Here's how the part is built. I have some questions about the finished solid (model axes, mm). Face numbers are marked on the shaded views. A direction names the side the tool comes from. Round coordinates to 2 decimals unless told otherwise and drop trailing zeros. Write each loop counter-clockwise with the first axis right and the second up, starting at its lowest first coordinate (ties: lowest second). Pieces come first, ordered by that corner, then holes. Notation, with made-up numbers: (84, 73.25) -> (135, 73.25) arc R24 ccw to (135, 85.25) -> close; hole circle Ø2 at (88.25, 2.25). An arc over 180 degrees is marked (long way). Put each result on its own line as item: value. Start each with the question number.
1. We'd pull the mould along X, two halves only. Please class the marked faces 1, 2 and 3: +X half, -X half, draft (parallel to the pull), parting line (faces both ways), or undercut.
2. I need wall thicknesses on probe 1 along X at (y, z) = (-0.95, 0.7); probe 2 along Z at (x, y) = (-1.75, -0.1). Which ranges of each line are inside material? Lowest first, please. Write a range as from..to.
3. Suppose I cut it at B-B (x = 1.5). Please give me the cut outline in (y, z), then the cut area to 3 significant figures.
4. Which directions (+Z, -Z, +X, -X, +Y, -Y) give clear straight access to the entire face, cutting with the end or side of a thin tool? Please do the marked faces 4, 5, 6, 7 and 8.
5. Suppose I cut it at D-D (x = -3.25). Please give me the cut outline in (y, z).
6. For pin 1 (0.7 mm diameter, centred on x = -3.5, y = 0, fed in from -Z); pin 2 (1.6 mm diameter, centred on x = -3, z = -0.5, fed in from +Y); pin 3 (1.5 mm diameter, centred on x = -0.5, z = 0, fed in from +Y), each with a flat end and sliding along its axis, tell me the tip position at first contact or that it passes through.
7. Suppose I cut it at A-A (z = 0). Please give me the cut outline in (x, y), then the cut area to 3 significant figures.
Autodesk Inventor part; units mm, degrees
ref_plane "Work Plane1" through (3, -0.7, -0.9) normal (1, 0, 0) x (0, 0, -1)
ref_plane "Work Plane2" through (-2, -0.7, 0.9) normal (-1, 0, 0) x (0, 0, 1)
ref_plane "YZ Plane" through (0, 0, 0) normal (1, 0, 0) x (0, 1, 0)
sketch "Sketch1" plane through (0, 0, 0) normal (0, 0, 1) x (1, 0, 0)
  circle A0 centre (0, 0) radius 0.6
  dimension "d0" = 1.2
extrude "Extrusion1" add sketch "Sketch1" against normal mid plane 6
sketch "Sketch3" plane through (0, 0, 0) normal (0, 0, 1) x (1, 0, 0)
  line L0 (0, 0) -> (3, 0)
  line L1 (0, 0) -> (-2, 0)
  line L2 (-2, 0) -> (-2, 0.9)
  line L3 (3, 0) -> (3, -0.9)
  line L4 (-2, 0.9) -> (3, 0.9)
  line L5 (3, 0.9) -> (3, -0.9)
  line L6 (3, -0.9) -> (-2, -0.9)
  line L7 (-2, -0.9) -> (-2, 0.9)
  dimension "d4" = 3
  dimension "d5" = 2
  dimension "d6" = 0.9
  dimension "d7" = 0.9
extrude "Extrusion2" add sketch "Sketch3" along normal mid plane 1.8
fillet "Fillet1" radius 0.2 4 edges at (0.5, 0.9, 0.9) (0.5, -0.9, 0.9) (0.5, 0.9, -0.9) (0.5, -0.9, -0.9)
ref_plane "Work Plane1" through (3, -0.7, -0.9) normal (1, 0, 0) x (0, 0, -1)
sketch "Sketch4" plane through (3, -0.7, -0.9) normal (1, 0, 0) x (0, 0, -1)
  circle A0 centre (-0.9, 0.7) radius 2.5
  dimension "d12" = 5
extrude "Extrusion3" add sketch "Sketch4" along normal blind 1
ref_plane "Work Plane2" through (-2, -0.7, 0.9) normal (-1, 0, 0) x (0, 0, 1)
sketch "Sketch5" plane through (-2, -0.7, 0.9) normal (-1, 0, 0) x (0, 0, 1)
  line L0 (-2.1, -0.6) -> (0.3, -0.6)
  line L1 (0.3, -0.6) -> (0.3, 2)
  line L2 (0.3, 2) -> (-2.1, 2)
  line L3 (-2.1, 2) -> (-2.1, -0.6)
  line L4 (-2.1, -0.6) -> (0.3, 2) construction
  line L5 (0.3, -0.6) -> (-2.1, 2) construction
  point P0 (-0.9, 0.7)
  dimension "d16" = 2.4
  dimension "d17" = 2.6
extrude "Extrusion4" add sketch "Sketch5" along normal blind 3
fillet "Fillet2" radius 0.2 12 edges at (-2, -1.3, 0) (-3.5, -1.3, -1.2) (-2, 0, -1.2) (-5, 0, -1.2) (-5, -1.3, 0) (-3.5, -1.3, 1.2) (-5, 0, 1.2) (-5, 1.3, 0) (-3.5, 1.3, 1.2) (-3.5, 1.3, -1.2) (-2, 1.3, 0) (-2, 0, 1.2)
fillet "Fillet3" radius 0.1 3 edges at (4, 0, 2.5) (-0.6, 0, 3) (-0.6, 0, -3)
properties part number "New_ThinGripper_base"
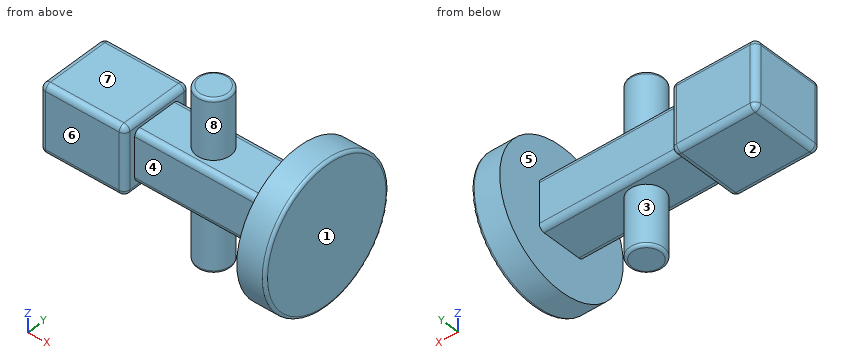
Verdict:
1. face 1: +X half
1. face 2: draft
1. face 3: undercut
2. probe 1: x = -5..-2, 3..4
2. probe 2: z = -0.9..0.9
3. outline: (-0.9, -0.7) arc R0.2 ccw to (-0.7, -0.9) -> (0.7, -0.9) arc R0.2 ccw to (0.9, -0.7) -> (0.9, 0.7) arc R0.2 ccw to (0.7, 0.9) -> (-0.7, 0.9) arc R0.2 ccw to (-0.9, 0.7) -> close
3. area: 3.21 mm^2
4. face 4: +Z, -Z, -Y
4. face 5: none
4. face 6: +Z, -Z, -X, -Y
4. face 7: +Z, -X, +Y, -Y
4. face 8: +Z
5. outline: (-1.3, -1) arc R0.2 ccw to (-1.1, -1.2) -> (1.1, -1.2) arc R0.2 ccw to (1.3, -1) -> (1.3, 1) arc R0.2 ccw to (1.1, 1.2) -> (-1.1, 1.2) arc R0.2 ccw to (-1.3, 1) -> close
6. pin 1: stops at z = -1.2
6. pin 2: stops at y = 1.3
6. pin 3: stops at y = 0.9
7. outline: (-5, -1.1) arc R0.2 ccw to (-4.8, -1.3) -> (-2.2, -1.3) arc R0.2 ccw to (-2, -1.1) -> (-2, -0.9) -> (3, -0.9) -> (3, -2.5) -> (3.9, -2.5) arc R0.1 ccw to (4, -2.4) -> (4, 2.4) arc R0.1 ccw to (3.9, 2.5) -> (3, 2.5) -> (3, 0.9) -> (-2, 0.9) -> (-2, 1.1) arc R0.2 ccw to (-2.2, 1.3) -> (-4.8, 1.3) arc R0.2 ccw to (-5, 1.1) -> close
7. area: 21.8 mm^2
